Can you work these out from the model? Positions are in its coordinate system, mm. Face numbers are marked on the shaded views. A direction names the side the tool comes from. Coordinates: 2 decimals unless noted, no trailing zeros. Write each loop counter-clockwise with the first axis right and the second up, starting at its lowest first coordinate (ties: lowest second). Pieces come first, ordered by that corner, then holes. Notation, with made-up numbers: M -4.75,11 L 21.25,11 A34 ccw 21.25,41 Z; hole C 86.5,44 d10. An arc over 180 degrees is marked long. Answer as a JSON object with one key per item and string values. Group by question number.
from build123d import *

# Parameters (mm, degrees)
SKETCH1_R                        = 7.5
BOSS_EXTRUDE1_DEPTH              = 7
SKETCH2_R                        = 12.8
BOSS_EXTRUDE2_DEPTH              = 5
SKETCH3_R                        = 2.5
CUT_EXTRUDE1_DEPTH               = 22.718195137
TAP_DRILL_FOR_M3X0_5_TAP1_REACH  = 27.631
TAP_DRILL_FOR_M3X0_5_TAP1_BORE_R = 1.3


with BuildPart() as part:
    # Sketch1 → Boss-Extrude1 (new body)
    with BuildSketch(Plane.XY):
        Circle(SKETCH1_R)
    extrude(amount=BOSS_EXTRUDE1_DEPTH)

    # Sketch2 → Boss-Extrude2 (add)
    with BuildSketch(Plane.XY.offset(7)):
        Circle(SKETCH2_R)
    extrude(amount=BOSS_EXTRUDE2_DEPTH)

    # Sketch3 → Cut-Extrude1 (cut, through all)
    with BuildSketch(Plane.XY.offset(12)):
        Circle(SKETCH3_R)
    extrude(amount=-CUT_EXTRUDE1_DEPTH, mode=Mode.SUBTRACT)

    # Tap Drill for M3x0.5 Tap1 bore (on position points) → Tap Drill for M3x0.5 Tap1 (cut, up to next)
    with BuildSketch(Plane(origin=(0, 7.5, 3), x_dir=(1, 0, 0), z_dir=(0, 1, 0)), mode=Mode.PRIVATE) as tap_drill_for_m3x0_5_tap1_sk1:
        Circle(TAP_DRILL_FOR_M3X0_5_TAP1_BORE_R)
    tap_drill_for_m3x0_5_tap1_tool1 = extrude(tap_drill_for_m3x0_5_tap1_sk1.sketch, amount=-TAP_DRILL_FOR_M3X0_5_TAP1_REACH, mode=Mode.PRIVATE) & part.part
    add(tap_drill_for_m3x0_5_tap1_tool1.solids().sort_by_distance((0, 7.5, 3))[0], mode=Mode.SUBTRACT)


solid = part.part
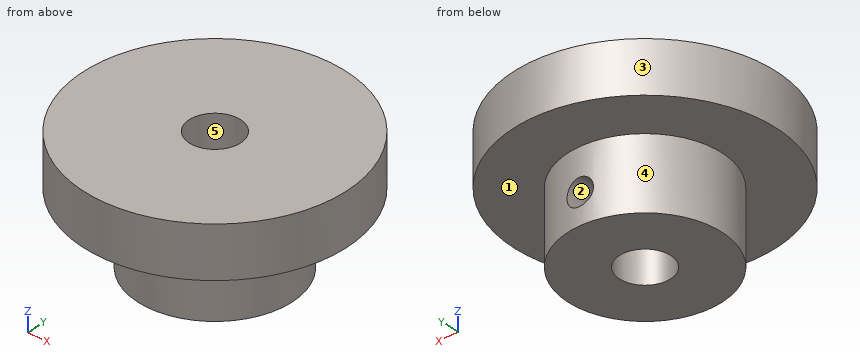
Q1. Please list where these lines run through material, in increasing order: L1, parallel to Y at x = 0, z = 7.5; L2, parallel to Z at x = 0, y = 4.65; L3, parallel to Z at x = 9.25, y = -4.5.
Q2. If we section it at C-C on z = 9.5: List the corners of the cut face in (x, y) for me.
Q3. If we section it at D-D on y = -3.75: List the corners of the cut face in (x, z) for me.
Q4. We'd pull the mould along X, two halves only. Please class the marked faces 1, 2 and 3: pulls with the +X half, pulls with the -X half, needs draft (parallel to the pull), parting line crosses it, or undercut.
Q5. On a 3-axis mill with a long thin cutter (end or side, diameter ignored), from which of +Z, -Z, +X, -X, +Y, -Y can I reach the whole of each face in a straight line? I mean the marked faces 4 and 5. Say none if no direction works.
Q6. Will these pins go through, and if not, where does the flat tip stop? pin 1 (13 mm diameter, centred on x = -4.5, y = 4.5, fed in from -Z); pin 2 (5 mm diameter, centred on x = -8, z = 8, fed in from +Y); pin 3 (4 mm diameter, centred on x = 0, y = 0, fed in from +Z); pin 4 (3 mm diameter, centred on x = -8, y = -8.5, fed in from -Z).
Q7. If we section it at B-B on x = 0: List the corners of the cut face in (y, z) for me, and give its area (3 significant figures).
Q8. If we section it at A-A on y = 0: List the corners of the cut face in (x, z) for me.
Reply:
{
 "1": {"L1": "-12.8 to -2.5, 2.5 to 12.8", "L2": "0 to 1.7, 4.3 to 12", "L3": "7 to 12"},
 "2": {"outline": "C 0,0 d25.6; hole C 0,0 d5"},
 "3": {"outline": "M -12.24,7 L -6.5,7 L -6.5,0 L 6.5,0 L 6.5,7 L 12.24,7 L 12.24,12 L -12.24,12 Z"},
 "4": {"face 1": "needs draft", "face 2": "undercut", "face 3": "parting line crosses it"},
 "5": {"face 4": "-Z", "face 5": "+Z, -Z"},
 "6": {"pin 1": "z = 0", "pin 2": "y = 11.56", "pin 3": "through", "pin 4": "z = 7"},
 "7": {"outline": "M -12.8,7 L -7.5,7 L -7.5,0 L -2.5,0 L -2.5,12 L -12.8,12 Z; M 2.5,0 L 7.5,0 L 7.5,1.7 L 2.5,1.7 Z; M 2.5,4.3 L 7.5,4.3 L 7.5,7 L 12.8,7 L 12.8,12 L 2.5,12 Z", "area": "160 mm^2"},
 "8": {"outline": "M -12.8,7 L -7.5,7 L -7.5,0 L -2.5,0 L -2.5,12 L -12.8,12 Z; M 2.5,0 L 7.5,0 L 7.5,7 L 12.8,7 L 12.8,12 L 2.5,12 Z"}
}
